Design review of the part built by this model. Coordinates are the model's own, in mm. A direction names the side the tool comes from. Coordinates: 2 decimals unless noted, no trailing zeros. Order: outer loops, then holes, each group sorted by start corner. A loop starts at its lowest first (then second) coordinate and runs counter-clockwise, first axis right, second up. Notation, with made-up numbers: (32.5, 68) -> (46.5, 68) arc R16 ccw to (46.5, 95) -> close; hole circle Ø7 at (43.5, 9). An arc over 180 degrees is marked (long way). Write item = value, one per line.
```python
from build123d import *

# Parameters (mm, degrees)
F0_W     = 101.6
F0_H     = 50.8
F1_DEPTH = 914.4
F2_W     = 25.4
F2_H     = 101.6
F3_DEPTH = 101.601
F4_R     = 3.175
F5_DEPTH = 50.801


with BuildPart() as f1:
    # F0 (on Top) → F1 (new body)
    with BuildSketch(Plane.XY):
        Rectangle(F0_W, F0_H)
    extrude(amount=F1_DEPTH)

    # F2 (on face) → F3 (cut, through all)
    with BuildSketch(Plane.YZ.offset(50.8)):
        with Locations((12.7, 457.2)):
            Rectangle(F2_W, F2_H)
        with Locations((12.7, 50.8)):
            Rectangle(F2_W, F2_H)
        with Locations((12.7, 863.6)):
            Rectangle(F2_W, F2_H)
    extrude(amount=-F3_DEPTH, mode=Mode.SUBTRACT)

    # F4 (on face) → F5 (cut, through all)
    with BuildSketch(Plane.XZ.offset(25.4)):
        with Locations((-25.4, 863.6)):
            Circle(F4_R)
        with Locations((-25.4, 457.2)):
            Circle(F4_R)
        with Locations((-25.4, 50.8)):
            Circle(F4_R)
        with Locations((25.4, 863.6)):
            Circle(F4_R)
        with Locations((25.4, 457.2)):
            Circle(F4_R)
        with Locations((25.4, 50.8)):
            Circle(F4_R)
    extrude(amount=-F5_DEPTH, mode=Mode.SUBTRACT)


solid = f1.part
```
(1) For faces 4 (the flat face through (1, 13, 508)), 5 (the flat face through (1, 13, 101.6)), 6 (the flat face through (1, 0, 863)), 7 (the flat face through (-1, -25.4, 451)), 8 (the flat face through (-1, 25.4, 252)), list the 3-axis set-ups (+Z, -Z, +X, -X, +Y, -Y) from which the entire face can be reached by the end or side of a thin tool; tool diameter is ignored.
Report:
face_4 = +X, -X, +Y
face_5 = -Z, +X, -X, +Y
face_6 = +Z, +X, -X, +Y
face_7 = +Z, -Z, +X, -X, -Y
face_8 = +Z, -Z, +X, -X, +Y
(2) We need section A-A (y = 10). Write out the cut boundary in (x, z), and give its area (3 significant figures).
Report:
outline = (-50.8, 101.6) -> (50.8, 101.6) -> (50.8, 406.4) -> (-50.8, 406.4) -> close; (-50.8, 508) -> (50.8, 508) -> (50.8, 812.8) -> (-50.8, 812.8) -> close
area = 61,900 mm²
(3) For L1, parallel to X at y = -19, z = 50; L2, parallel to Z at x = -25.4, y = -12.75 (3 decimals); L3, parallel to Z at x = -25, y = -6, list the stretches that pass through material, from the lowest coordinate up.
Report:
L1 = -50.8 to -28.47, -22.33 to 22.33, 28.47 to 50.8
L2 = 0 to 47.625, 53.975 to 454.025, 460.375 to 860.425, 866.775 to 914.4
L3 = 0 to 47.65, 53.95 to 454.05, 460.35 to 860.45, 866.75 to 914.4
(4) The part is to be moulded in two halves that separate along Z. For faces 1 (the flat face through (1, 13, 406.4)), 2 (the flat face through (-1, -13, 914.4)), 3 (the flat face through (50.8, -0.4, 450.8)), say which applies: released by +Z, released by -Z, zero draft, split by the parting line, or undercut.
Report:
face_1 = undercut
face_2 = released by +Z
face_3 = zero draft
(5) We need section B-B (x = 14). Write out the cut boundary in (y, z).
Report:
outline = (-25.4, 0) -> (0, 0) -> (0, 101.6) -> (25.4, 101.6) -> (25.4, 406.4) -> (0, 406.4) -> (0, 508) -> (25.4, 508) -> (25.4, 812.8) -> (0, 812.8) -> (0, 914.4) -> (-25.4, 914.4) -> close
(6) Insertion check: pin 1 (5.5 mm diameter, centred on x = 25.4, z = 457.2, fed in from +Y); pin 2 (12.5 mm diameter, centred on x = 21.5, y = 14.5, fed in from +Z); pin 3 (7.5 mm diameter, centred on x = -25.4, z = 457.2, fed in from +Y); pin 4 (6 mm diameter, centred on x = -15.5, y = 12.5, fed in from -Z). Each pin has a flat end and moves straight along its axis. Give the tip position at first contact, or say it passes through.
Report:
pin_1 = through
pin_2 = 812.8
pin_3 = 0
pin_4 = 101.6
